Model file for the job. Use its own axes, mm. A direction names the side the tool comes from. Round coordinates to 2 decimals unless told otherwise and drop trailing zeros. Loops run counter-clockwise (first coordinate to the right, second up) from the corner with the lowest first, then second, coordinate; pieces in that order, holes last. Notation, with made-up numbers: (25.25, 58) -> (30.25, 58) arc R16 ccw to (30.25, 85) -> close; hole circle Ø2 at (32, -4). An arc over 180 degrees is marked (long way). Use a Markdown table: item, result.
from build123d import *

# Parameters (mm, degrees)
F0_W      = 14
F0_H      = 8
F1_DEPTH  = 6
F3_DEPTH  = 25
F5_DEPTH  = 15
F6_R      = 0.5
F7_W      = 6
F7_H      = 6
F8_DEPTH  = 2.5
F10_DEPTH = 25


with BuildPart() as f1:
    # F0 (on Top) → F1 (new body)
    with BuildSketch(Plane.XY):
        Rectangle(F0_W, F0_H)
    extrude(amount=F1_DEPTH)

    # F2 (on face) → F3 (cut, symmetric)
    with BuildSketch(Plane(origin=(-7, 0, 0), x_dir=(0, -1, 0), z_dir=(-1, 0, 0))):
        with BuildLine():
            Line((-2.8831406487, 6), (2.8831406487, 6))
            ThreePointArc((2.8831406487, 6), (0, 7.75), (-2.8831406487, 6))
        make_face()
        with BuildLine():
            ThreePointArc((-2.8831406487, 6), (-0.7721052039, 1.3430467925), (3.25, 4.5))
            ThreePointArc((3.25, 4.5), (3.1569532075, 5.2721052039), (2.8831406487, 6))
            Line((2.8831406487, 6), (-2.8831406487, 6))
        make_face()
    extrude(amount=F3_DEPTH, both=True, mode=Mode.SUBTRACT)

    # F4 (on face) → F5 (cut, symmetric)
    with BuildSketch(Plane(origin=(-7, 0, 0), x_dir=(0, -1, 0), z_dir=(-1, 0, 0))):
        with BuildLine():
            Line((8.3296196082, 2), (8.3296196082, 11.0180403529))
            Line((8.3296196082, 11.0180403529), (-8.3296196082, 11.0180403529))
            Line((-8.3296196082, 11.0180403529), (-8.3296196082, 2))
            Line((-8.3296196082, 2), (-4, 2))
            Line((-4, 2), (-4, 6))
            Line((-4, 6), (-2.8831406487, 6))
            ThreePointArc((-2.8831406487, 6), (-3.1858900819, 3.8576571119), (-2.0766559657, 2))
            Line((-2.0766559657, 2), (2.0766559657, 2))
            ThreePointArc((2.0766559657, 2), (3.1858900819, 3.8576571119), (2.8831406487, 6))
            Line((2.8831406487, 6), (4, 6))
            Line((4, 6), (4, 2))
            Line((4, 2), (8.3296196082, 2))
        make_face()
        with BuildLine():
            Line((-4, 6), (-4, 2))
            Line((-4, 2), (-2.0766559657, 2))
            ThreePointArc((-2.0766559657, 2), (-3.1858900819, 3.8576571119), (-2.8831406487, 6))
            Line((-2.8831406487, 6), (-4, 6))
        make_face()
        with BuildLine():
            Line((2.0766559657, 2), (4, 2))
            Line((4, 2), (4, 6))
            Line((4, 6), (2.8831406487, 6))
            ThreePointArc((2.8831406487, 6), (3.1858900819, 3.8576571119), (2.0766559657, 2))
        make_face()
    extrude(amount=F5_DEPTH, both=True, mode=Mode.SUBTRACT)

    # F6
    f6_edges = [f1.edges().sort_by_distance(p)[0] for p in [
        (0, 4, 2),
        (0, 2.076656, 2),
        (0, -2.076656, 2),
        (0, -4, 2),
    ]]
    fillet(f6_edges, radius=F6_R)

    # F7 (on Right) → F8 (join, symmetric)
    with BuildSketch(Plane.YZ):
        with Locations((0, 3)):
            Rectangle(F7_W, F7_H)
    extrude(amount=F8_DEPTH, both=True)

    # F9 (on face) → F10 (cut)
    with BuildSketch(Plane(origin=(-2.5, 0, 0), x_dir=(0, -1, 0), z_dir=(-1, 0, 0))):
        with BuildLine():
            Line((-1.3447056541, 5.2670448107), (-1, 4.4))
            ThreePointArc((-1, 4.4), (0, 3.4), (1, 4.4))
            ThreePointArc((1, 4.4), (0.7071067812, 5.1071067812), (0, 5.4))
            Line((0, 5.4), (0, 6))
            Line((0, 6), (-3, 6))
            Line((-3, 6), (-3, 2))
            Line((-3, 2), (-2.25, 2))
            ThreePointArc((-2.25, 2), (-2.091886117, 1.974341649), (-1.95, 1.9))
            Line((-1.95, 1.9), (-1.6, 3.035565484))
            Line((-1.6, 3.035565484), (-1.6, 4.4))
            Line((-1.6, 4.4), (-1.6, 5.2670448107))
            Line((-1.6, 5.2670448107), (-1.3447056541, 5.2670448107))
        make_face()
        with BuildLine():
            ThreePointArc((0, 6), (1.1313708499, 5.5313708499), (1.6, 4.4))
            Line((1.6, 4.4), (1.6, 3.035565484))
            Line((1.6, 3.035565484), (1.95, 1.9))
            ThreePointArc((1.95, 1.9), (2.091886117, 1.974341649), (2.25, 2))
            Line((2.25, 2), (3, 2))
            Line((3, 2), (3, 6))
            Line((3, 6), (0, 6))
        make_face()
    extrude(amount=-F10_DEPTH, mode=Mode.SUBTRACT)


solid = f1.part
Q1. Band-saw the part on D-D, the plane z = 5.6. Give the cut face in (x, y), plus the area to 3 significant figures.
Results list:
| item | result |
|---|---|
| outline | (-2.5, -1.06) -> (2.5, -1.06) -> (2.5, 0) -> (-2.5, 0) -> close |
| area | 5.29 mm² |
Q2. Band-saw the part on C-C, the plane x = -2. Give the cut face in (y, z), plus the area to 3 significant figures.
Results list:
| item | result |
|---|---|
| outline | (-4, 0) -> (4, 0) -> (4, 1.5) arc R0.5 ccw to (3.5, 2) -> (2.25, 2) arc R0.5 ccw to (1.95, 1.9) -> (1.6, 3.04) -> (1.6, 5.27) -> (1.34, 5.27) -> (1, 4.4) arc R1 cw (long way) to (0, 5.4) -> (0, 6) arc R1.6 ccw to (-1.6, 4.4) -> (-1.6, 3.04) -> (-1.95, 1.9) arc R0.5 ccw to (-2.25, 2) -> (-3.5, 2) arc R0.5 ccw to (-4, 1.5) -> close |
| area | 23.9 mm² |
Q3. Band-saw the part on B-B, the plane y = -1.75. Give the cut face in (x, z).
Results list:
| item | result |
|---|---|
| outline | (-7, 0) -> (7, 0) -> (7, 1.76) -> (2.5, 1.76) -> (2.5, 2.55) -> (-2.5, 2.55) -> (-2.5, 1.76) -> (-7, 1.76) -> close |
Q4. Flat gauge pins, fed straight in: pin 1 (1.1 mm diameter, centred on x = 0, z = 4, fed in from +Y); pin 2 (2 mm diameter, centred on y = 1, z = 4, fed in from -X); pin 3 (2 mm diameter, centred on y = -0.5, z = 2.5, fed in from +X). Where does each tip first touch, or does it go through?
Results list:
| item | result |
|---|---|
| pin 1 | stops at y = 1.6 |
| pin 2 | stops at x = -2.5 |
| pin 3 | stops at x = 2.5 |
Q5. Band-saw the part on A-A, the plane x = -6. Give the cut face in (y, z), plus the area to 3 significant figures.
Results list:
| item | result |
|---|---|
| outline | (-4, 0) -> (4, 0) -> (4, 1.5) arc R0.5 ccw to (3.5, 2) -> (2.25, 2) arc R0.5 ccw to (1.95, 1.9) arc R3.25 cw to (-1.95, 1.9) arc R0.5 ccw to (-2.25, 2) -> (-3.5, 2) arc R0.5 ccw to (-4, 1.5) -> close |
| area | 13.8 mm² |
Q6. Tool access for faces 1 (the face through (2.5, 0, 3)), 2 (the face through (-2.5, 0, 3)), 3 (the face through (0, 1.6, 4)), 4 (the face through (0, -3, 2)): list every direction of +Z, -Z, +X, -X, +Y, -Y with a clear straight run to the whole face (end or side of a thin tool).
Results list:
| item | result |
|---|---|
| face 1 | +Z, +X |
| face 2 | +Z, -X |
| face 3 | +Z, +X, -X, +Y |
| face 4 | +Z, +X, -X, -Y |
Q7. Drill centre lines: L1, parallel to Z at x = -1, y = -3.25; L2, parallel to Z at x = -4.5, y = -1.25; L3, parallel to X at y = -1.5, z = 3.35. Where is each one in solid material? Low to high. Write a range as from..to.
Results list:
| item | result |
|---|---|
| L1 | z = 0..2 |
| L2 | z = 0..1.5 |
| L3 | x = -2.5..2.5 |
